from build123d import *

# Parameters (mm, degrees)
BOSS_EXTRUDE1_DEPTH      = 10
BOSS_EXTRUDE2_DEPTH      = 1.9
BOSS_EXTRUDE2_DEPTH_BACK = 1.9
SKETCH2_R                = 3.5
SKETCH3_R                = 4
CUT_EXTRUDE1_DEPTH       = 39.727380495
SKETCH4_R                = 4
CUT_EXTRUDE2_DEPTH       = 39.727380495
SKETCH5_R                = 1.2
CUT_EXTRUDE3_DEPTH       = 3.8
SKETCH9_W                = 19.801856387
SKETCH9_H                = 10
CUT_EXTRUDE4_DEPTH       = 1
SKETCH12_W               = 14.5
SKETCH12_H               = 5.5
BOSS_EXTRUDE3_DEPTH      = 3
BOSS_EXTRUDE3_TAPER      = 8
SKETCH10_R               = 2.25
CUT_EXTRUDE5_DEPTH       = 37.680126397
FILLET1_R                = 2
FILLET2_R                = 1
CUT_EXTRUDE7_DEPTH       = 7.342905


# Read off the part's stored shape, not the designer's step: Boss-Extrude4
with BuildPart() as part:
    # Sketch1 → Boss-Extrude1 (new body)
    with BuildSketch(Plane.XY):
        with BuildLine():
            Line((-15.093376031, -5), (-32.8, -13.865042807))
            Line((-32.8, -13.865042807), (-3.400702634, -19.099613127))
            ThreePointArc((-3.400702634, -19.099613127), (12.457655656, -14.871678303), (19.4, 0))
            Line((19.4, 0), (15.9, 0))
            ThreePointArc((15.9, 0), (2.532323154, -15.697048749), (-15.093376031, -5))
        make_face()
    extrude(amount=BOSS_EXTRUDE1_DEPTH)

    # Sketch2 → Boss-Extrude2 (add, two sides: drawn at the far end of the back side and taken through both)
    with BuildSketch(Plane.XY.offset(5).offset(-BOSS_EXTRUDE2_DEPTH_BACK)):
        with Locations((19.4, 0)):
            Circle(SKETCH2_R)
    extrude(amount=BOSS_EXTRUDE2_DEPTH + BOSS_EXTRUDE2_DEPTH_BACK)

    # Sketch3 → Cut-Extrude1 (cut, through all)
    with BuildSketch(Plane.XY.offset(6.9)):
        with Locations((19.4, 0)):
            Circle(SKETCH3_R)
    extrude(amount=CUT_EXTRUDE1_DEPTH, mode=Mode.SUBTRACT)

    # Sketch4 → Cut-Extrude2 (cut, through all)
    with BuildSketch(Plane(origin=(0, 0, 3.1), x_dir=(-1, 0, 0), z_dir=(0, 0, -1))):
        with Locations((-19.4, 0)):
            Circle(SKETCH4_R)
    extrude(amount=CUT_EXTRUDE2_DEPTH, mode=Mode.SUBTRACT)

    # Sketch5 → Cut-Extrude3 (cut)
    with BuildSketch(Plane(origin=(0, 0, 3.1), x_dir=(-1, 0, 0), z_dir=(0, 0, -1))):
        with Locations((-19.4, 0)):
            Circle(SKETCH5_R)
    extrude(amount=-CUT_EXTRUDE3_DEPTH, mode=Mode.SUBTRACT)

    # Sketch9 → Cut-Extrude4 (cut)
    with BuildSketch(Plane(origin=(-1.023487263, 2.044265831, 0), x_dir=(0.8941901013439871, 0.4476874609126664, 0), z_dir=(-0.4476874609126664, 0.8941901013439871, 0))):
        with Locations((-25.63571294, -5)):
            Rectangle(SKETCH9_W, SKETCH9_H)
    extrude(amount=-CUT_EXTRUDE4_DEPTH, mode=Mode.SUBTRACT)

    # Sketch12 → Boss-Extrude3 (add)
    with BuildSketch(Plane(origin=(-0.575799802, 1.15007573, 0), x_dir=(0.894190101343987, 0.44768746091266626, 0), z_dir=(-0.4476874609126663, 0.8941901013439871, 0))):
        with Locations((-25.74136864, -5)):
            Rectangle(SKETCH12_W, SKETCH12_H)
    extrude(amount=BOSS_EXTRUDE3_DEPTH, taper=BOSS_EXTRUDE3_TAPER)

    # Boss-Extrude4 outline → Boss-Extrude4 (revolve)
    with BuildSketch(Plane(origin=(-22.3, 0, 5), x_dir=(1, 0, 0), z_dir=(0, 0, 1))):
        Polygon((0, -10), (3.25, -10), (2.968804119, -4.634462949), (0, -4.634462949), align=None)
    revolve(axis=Axis((-22.3, 0, 5), (0, 1, 0)))

    # Sketch10 → Cut-Extrude5 (cut, through all)
    with BuildSketch(Plane(origin=(-1.672257199, 0, 0), x_dir=(1, 0, 0), z_dir=(0, -1, 0))):
        with Locations(Location((-20.627742801, 5, 0), (0, 0, 90))):
            Circle(SKETCH10_R)
    extrude(amount=CUT_EXTRUDE5_DEPTH, mode=Mode.SUBTRACT)

    # Fillet1
    fillet1_edges = [part.edges().sort_by_distance(p)[0] for p in [
        (18.987628866, -3.978686975, 8.45),
        (18.987628866, -3.978686975, 1.55),
        (-14.746830764, -5.944828206, 5),
    ]]
    fillet(fillet1_edges, radius=FILLET1_R)

    # Fillet2
    fillet2_edges = [part.edges().sort_by_distance(p)[0] for p in [
        (15.803350515, -1.750460649, 8.45),
        (15.803350515, -1.750460649, 1.55),
    ]]
    fillet(fillet2_edges, radius=FILLET2_R)

    # Sketch15 → Cut-Extrude7 (cut)
    with BuildSketch(Plane(origin=(0, -20, 0), x_dir=(1, 0, 0), z_dir=(0, 1, 0))):
        Polygon((-19.066838493, -5), (-20.683419246, -2.2), (-23.916580754, -2.2), (-25.533161507, -5), (-23.916580754, -7.8), (-20.683419246, -7.8), align=None)
    extrude(amount=CUT_EXTRUDE7_DEPTH, mode=Mode.SUBTRACT)


solid = part.part
Geometry: final body of the model. Coordinates: model frame, mm. A direction names the side the tool comes from. Coordinates: 2 decimals unless noted, no trailing zeros. Order: outer loops, then holes, each group sorted by start corner. A loop starts at its lowest first (then second) coordinate and runs counter-clockwise, first axis right, second up.
(1) Section query C-C (x = -6). Return the cut outline in (y, z).
(2) Material intervals for probe 1 along Y at (x, z) = (19.4, 5.95); probe 2 along X at (y, z) = (-9.25, 5); probe 3 along X at (y, z) = (-7, 5.75), sorted ascending.
(3) Access query for faces 1 (the face through (22.062, 2.272, 4.973)), 2 (the face through (-22, -14, 2.2)), 3 (the face through (-24, -4.634, 3)). Directions: +Z, -Z, +X, -X, +Y, -Y. A direction counts if a zero-diameter tool reaches every point of the face in a straight line with its end or side. Return the directions, or none.
(4) Section query A-A (x = 20). Return the cut outline in (y, z), plus the area to 3 significant figures.
(5) Section query B-B (y = -11.25). State how many separate pieces and enclosed holes the cut face has, plus the area to 3 significant figures.
(6) Draft query along Z for faces 4 (the face through (-6, -15, 10)), 5 (the face through (-20, -12.657, 6)), 6 (the face through (18.29, -0.46, 4.97)). Return one class per face: pulls with the +Z half, pulls with the -Z half, needs draft (parallel to the pull), parting line crosses it, or undercut.
(7) Section query D-D (x = 5). Return the cut outline in (y, z).
(8) First-contact query: pin 1 (4 mm diameter, centred on x = 10, z = 6.5, fed in from +Y); pin 2 (3 mm diameter, centred on x = -15.5, z = 1.5, fed in from -Y); pin 3 (12 mm diameter, centred on x = -23.5, y = -1.5, fed in from +Z). Flat tips, straight axial feed; report the tip coordinate or a pass-through.
Solution:
1. outline: (-18.64, 0) - (-14.72, 0) - (-14.72, 10) - (-18.64, 10) - close
2. probe 1: y = -3.5 to -1.2, 1.2 to 3.5
2. probe 2: x = -28.05 to -24.55, -20.05 to -12.93, 12.93 to 17.05
2. probe 3: x = -25.3 to -24.42, -20.18 to -17.2, -16.85 to -14.54, 14.28 to 18.09
3. face 1: +Z, -Z
3. face 2: -Y
3. face 3: +Z, -Z, -X, +Y
4. outline: (-3.45, 3.1) - (-1.04, 3.1) - (-1.04, 6.9) - (-3.45, 6.9) - close; (1.04, 3.1) - (3.45, 3.1) - (3.45, 6.9) - (1.04, 6.9) - close
4. area: 18.3 mm2
5. separate pieces: 2
5. enclosed holes: 1
5. area: 199 mm2
6. face 4: pulls with the +Z half
6. face 5: undercut
6. face 6: needs draft
7. outline: (-18.74, 0) - (-15.09, 0) - (-15.09, 10) - (-18.74, 10) - close
8. pin 1: stops at y = -10.43
8. pin 2: stops at y = -17.21
8. pin 3: stops at z = 8.11
